from build123d import *

# Parameters (mm, degrees)
SKETCH1_W           = 10
SKETCH1_H           = 5
SKETCH1_W_2         = 25
SKETCH1_W_3         = 20
BOSS_EXTRUDE1_DEPTH = 5
SKETCH2_W           = 5
SKETCH2_H           = 5
CUT_EXTRUDE1_DEPTH  = 1


with BuildPart() as part:
    # Sketch1 → Boss-Extrude1 (new body)
    with BuildSketch(Plane.XY):
        Polygon((-20, 0), (0, 0), (0, 12), (-20, 12), (-40, 12), (-50, 12), (-55, 12), (-65, 12), (-65, 0), (-40, 0), align=None)
        with Locations((-60, 14.5)):
            Rectangle(SKETCH1_W, SKETCH1_H)
        with Locations((-45, 14.5)):
            Rectangle(SKETCH1_W, SKETCH1_H)
        with Locations((-52.5, -2.5)):
            Rectangle(SKETCH1_W_2, SKETCH1_H)
        with Locations((-10, -2.5)):
            Rectangle(SKETCH1_W_3, SKETCH1_H)
        with Locations((-10, 14.5)):
            Rectangle(SKETCH1_W_3, SKETCH1_H)
    extrude(amount=BOSS_EXTRUDE1_DEPTH)

    # Sketch2 → Cut-Extrude1 (cut)
    with BuildSketch(Plane(origin=(-40, 0, 0), x_dir=(0, 0, -1), z_dir=(1, 0, 0))):
        with Locations((-2.5, 14.5)):
            Rectangle(SKETCH2_W, SKETCH2_H)
    extrude(amount=-CUT_EXTRUDE1_DEPTH, mode=Mode.SUBTRACT)


solid = part.part
Check sheet for the modelled part. Datum: model origin and axes. Units: mm. A direction names the side the tool comes from. Give positions to 0.01 mm unless a question says otherwise; leave off trailing zeros. Loops run counter-clockwise (first coordinate to the right, second up) from the corner with the lowest first, then second, coordinate; pieces in that order, holes last. Notation, with made-up numbers: M 45.25,-5.75 L 104.25,-5.75 A34 cw 104.25,30.25 Z; hole C 50,69 d8. An arc over 180 degrees is marked long. Answer as a JSON object with one key per item and string values. Group by question number.
Q1. Cross-section at B-B on z = 0.6. Record the cut outline in (x, y), then the cut area to 3 significant figures.
Q2. Cross-section at C-C on x = -25. Record the cut outline in (y, z), then the cut area to 3 significant figures.
Q3. Access from +Z, -Z, +X, -X, +Y, -Y to the whole of each face (thin tool, end or side, straight path). Record for faces 5 (the flat face through (0, 6, 2)), 6 (the flat face through (-40, -3, 2)), 7 (the flat face through (-55, 14, 2)).
Q4. Material ranges on line 1 along X through (y, z) = (12.25, 1.1); line 2 along Y through (x, z) = (-54.5, 4.5); line 3 along Y through (x, z) = (-37, 2.2), recorded low to high. Write a range as [from, to].
Q5. Cross-section at D-D on x = -54. Record the cut outline in (y, z).
Q6. Release check for a two-part mould opening along X. For faces 1 (the flat face through (-50, 14, 2)), 2 (the flat face through (-65, 6, 2)), 3 (the flat face through (-46, 17, 2)), 4 (the flat face through (-30, 12, 2)) record: released by +X, released by -X, zero draft, split by the parting line, or undercut.
Q7. Cross-section at A-A on y = -0.75. Record the cut outline in (x, z).
Q8. Go/stop test with flat-tipped pins: P1, Ø1.5, axis at y = 14.5, z = 1.5, coming from the +X side; P2, Ø1.5, axis at x = -31.5, z = 2, coming from the -Y side; P3, Ø1.5, axis at x = -28, z = 1.5, coming from the +Y side. Record where each tip stops, or that it passes through.
Evaluation:
{
 "1": {"outline": "M -65,-5 L -40,-5 L -40,0 L -20,0 L -20,-5 L 0,-5 L 0,17 L -20,17 L -20,12 L -41,12 L -41,17 L -50,17 L -50,12 L -55,12 L -55,17 L -65,17 Z", "area": "1,200 mm2"},
 "2": {"outline": "M 0,0 L 12,0 L 12,5 L 0,5 Z", "area": "60.0 mm2"},
 "3": {"face 5": "+Z, -Z, +X, +Y, -Y", "face 6": "+Z, -Z, -Y", "face 7": "+Z, -Z, +Y"},
 "4": {"line 1": "x = [-65, -55], [-50, -41], [-20, 0]", "line 2": "y = [-5, 12]", "line 3": "y = [0, 12]"},
 "5": {"outline": "M -5,0 L 12,0 L 12,5 L -5,5 Z"},
 "6": {"face 1": "undercut", "face 2": "released by -X", "face 3": "zero draft", "face 4": "undercut"},
 "7": {"outline": "M -65,0 L -40,0 L -40,5 L -65,5 Z; M -20,0 L 0,0 L 0,5 L -20,5 Z"},
 "8": {"P1": "stops at x = 0", "P2": "stops at y = 0", "P3": "stops at y = 12"}
}
